```python
from build123d import *

# Parameters (mm, degrees)
F1_DEPTH = 25.4


# Not quite as in the source:
# - a feature names something its author has since deleted; it is built from what else it names


with BuildPart() as f1:
    # F0 (on Front) → F1 (new body)
    with BuildSketch(Plane.XZ):
        with BuildLine():
            ThreePointArc((33.018049972, 14.6313424898), (30.0088601414, 17.9049378249), (26.6767187304, 20.8491666667))
            ThreePointArc((26.6767187304, 20.8491666667), (0, 65.0875), (-26.6767187304, 20.8491666667))
            ThreePointArc((-26.6767187304, 20.8491666667), (-30.0088601414, 17.9049378249), (-33.018049972, 14.6313424898))
            ThreePointArc((-33.018049972, 14.6313424898), (-41.8158398527, -3.2856787995), (-41.5452899235, -23.2443250813))
            ThreePointArc((-41.5452899235, -23.2443250813), (-35.8973631324, -36.1216401303), (-26.3860544261, -46.4782480018))
            ThreePointArc((-26.3860544261, -46.4782480018), (-18.6113486842, -51.3110295952), (-9.9877042304, -54.3826063299))
            ThreePointArc((-9.9877042304, -54.3826063299), (0, -55.5625), (9.9877042304, -54.3826063299))
            ThreePointArc((9.9877042304, -54.3826063299), (18.6113486842, -51.3110295952), (26.3860544261, -46.4782480018))
            ThreePointArc((26.3860544261, -46.4782480018), (35.8973631324, -36.1216401303), (41.5452899235, -23.2443250813))
            ThreePointArc((41.5452899235, -23.2443250813), (41.8158398527, -3.2856787995), (33.018049972, 14.6313424898))
        make_face()
        with BuildLine():
            ThreePointArc((20.4107142857, 47.190312821), (23.7132340956, 32.7529767549), (17.8428848253, 19.1558333333))
            ThreePointArc((17.8428848253, 19.1558333333), (0, -49.2125), (-17.8428848253, 19.1558333333))
            ThreePointArc((-17.8428848253, 19.1558333333), (-23.7132340956, 32.7529767549), (-20.4107142857, 47.190312821))
            ThreePointArc((-20.4107142857, 47.190312821), (-10.6767956636, 53.2964751512), (0, 49.0490730624))
            ThreePointArc((0, 49.0490730624), (10.6767956636, 53.2964751512), (20.4107142857, 47.190312821))
        make_face(mode=Mode.SUBTRACT)
        with BuildLine():
            ThreePointArc((31.7028005699, -58.996710055), (31.1832359324, -51.8291005513), (26.3860544261, -46.4782480018))
            ThreePointArc((26.3860544261, -46.4782480018), (18.6113486842, -51.3110295952), (9.9877042304, -54.3826063299))
            ThreePointArc((9.9877042304, -54.3826063299), (10.009677281, -58.0934630853), (11.2522370234, -61.5901738197))
            ThreePointArc((11.2522370234, -61.5901738197), (17.8174676094, -59.9971626047), (22.102310986, -65.220193776))
            ThreePointArc((22.102310986, -65.220193776), (24.9477521066, -59.0929266684), (31.7028005699, -58.996710055))
        make_face()
        with BuildLine():
            ThreePointArc((-9.9877042304, -54.3826063299), (-18.6113486842, -51.3110295952), (-26.3860544261, -46.4782480018))
            ThreePointArc((-26.3860544261, -46.4782480018), (-31.1832359324, -51.8291005513), (-31.7028005699, -58.996710055))
            ThreePointArc((-31.7028005699, -58.996710055), (-24.9477521066, -59.0929266684), (-22.102310986, -65.220193776))
            ThreePointArc((-22.102310986, -65.220193776), (-17.8174676094, -59.9971626047), (-11.2522370234, -61.5901738197))
            ThreePointArc((-11.2522370234, -61.5901738197), (-10.009677281, -58.0934630853), (-9.9877042304, -54.3826063299))
        make_face()
        with BuildLine():
            add(Edge.make_bspline(
                [(33.018049972, 14.6313424898), (46.9965733011, 11.8619536122), (150.360470689, -0.7954577234), (49.0987253283, -9.3555527531), (41.5452899235, -23.2443250813)],
                knots=[0, 0, 0, 0, 0.5108094749, 1, 1, 1, 1], degree=3))
            ThreePointArc((33.018049972, 14.6313424898), (41.8158398527, -3.2856787995), (41.5452899235, -23.2443250813))
        make_face()
        with BuildLine():
            ThreePointArc((-41.5452899235, -23.2443250813), (-41.8158398527, -3.2856787995), (-33.018049972, 14.6313424898))
            add(Edge.make_bspline(
                [(-33.018049972, 14.6313424898), (-46.9965733011, 11.8619536122), (-150.360470689, -0.7954577234), (-49.0987253283, -9.3555527531), (-41.5452899235, -23.2443250813)],
                knots=[0, 0, 0, 0, 0.5108094749, 1, 1, 1, 1], degree=3))
        make_face()
    extrude(amount=F1_DEPTH)


solid = f1.part
```
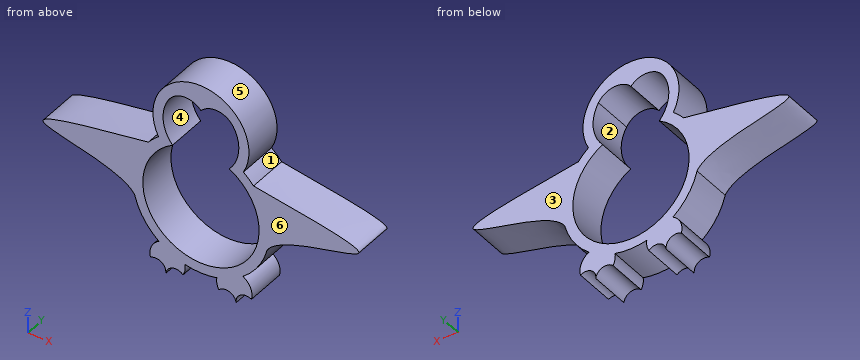
Input: part model. Units: mm. Frame: model coordinates. Face numbers are marked on the shaded views. A direction names the side the tool comes from. Coordinates: 2 decimals unless noted, no trailing zeros. Order: outer loops, then holes, each group sorted by start corner. A loop starts at its lowest first (then second) coordinate and runs counter-clockwise, first axis right, second up. Notation, with made-up numbers: (-5.75, 27) - (12.25, 27) arc R16 ccw to (12.25, 33) - close; hole circle Ø1 at (23, -31.5). An arc over 180 degrees is marked (long way). Return JSON: item names as keys, results as strings.
Q1. Access query for the marked faces 1, 2 and 3. Directions: +Z, -Z, +X, -X, +Y, -Y. A direction counts if a zero-diameter tool reaches every point of the face in a straight line with its end or side. Return the directions, or none.
The answers:
{"face 1": "+X, +Y, -Y", "face 2": "+Y, -Y", "face 3": "+Z, -Z, +X, -X, +Y"}
Q2. Draft query along X for the marked faces 4, 5 and 6. Return one class per face: +X half, -X half, draft (parallel to the pull), parting line (faces both ways), or undercut.
The answers:
{"face 4": "undercut", "face 5": "parting line", "face 6": "draft"}
Q3. First-contact query: pin 1 (1 mm diameter, centred on x = -5, y = -4.5, fed in from -Z); pin 2 (12 mm diameter, centred on y = -20, z = 24, fed in from +X); pin 3 (4 mm diameter, centred on y = -13, z = 40, fed in from -X). Flat tips, straight axial feed; report the tip coordinate or a pass-through.
The answers:
{"pin 1": "stops at z = -55.33", "pin 2": "stops at x = 29.91", "pin 3": "stops at x = -30.01"}
Q4. Ray query, probe 1 along Z at (x, y) = (18, -4.5); probe 2 along X at (y, z) = (-19.5, 39.5); probe 3 along X at (y, z) = (-16.75, -28.5). Return the intervals inside material, ascending.
The answers:
{"probe 1": "z = -60.06 to -44.47, 19.07 to 19.34, 50.11 to 59.13", "probe 2": "x = -29.81 to -23.37, 23.37 to 29.81", "probe 3": "x = -39.84 to -32.92, 32.92 to 39.84"}
Q5. Cut plane A-A (x = -4.5). Return loops of the section in (y, z), then the cut area to 3 significant figures.
The answers:
{"outline": "(-25.4, -55.33) - (0, -55.33) - (0, -48.93) - (-25.4, -48.93) - close; (-25.4, 52.31) - (0, 52.31) - (0, 64.75) - (-25.4, 64.75) - close", "area": "478 mm2"}
